Study the drawing (mm; zero at the part's minimum x, y, z) and answer. A direction names the side the tool comes from. Coordinates: 2 decimals unless noted, no trailing zeros. Loops run counter-clockwise (first coordinate to the right, second up) from the corner with the lowest first, then second, coordinate; pieces in that order, holes last. Notation, with made-up numbers: (4.25, -18) -> (57.25, -18) arc R24 cw to (57.25, 16) -> close; hole circle Ø6 at (-9.75, -34.75). An arc over 180 degrees is marked (long way). One line per question, with ' | ' between items.
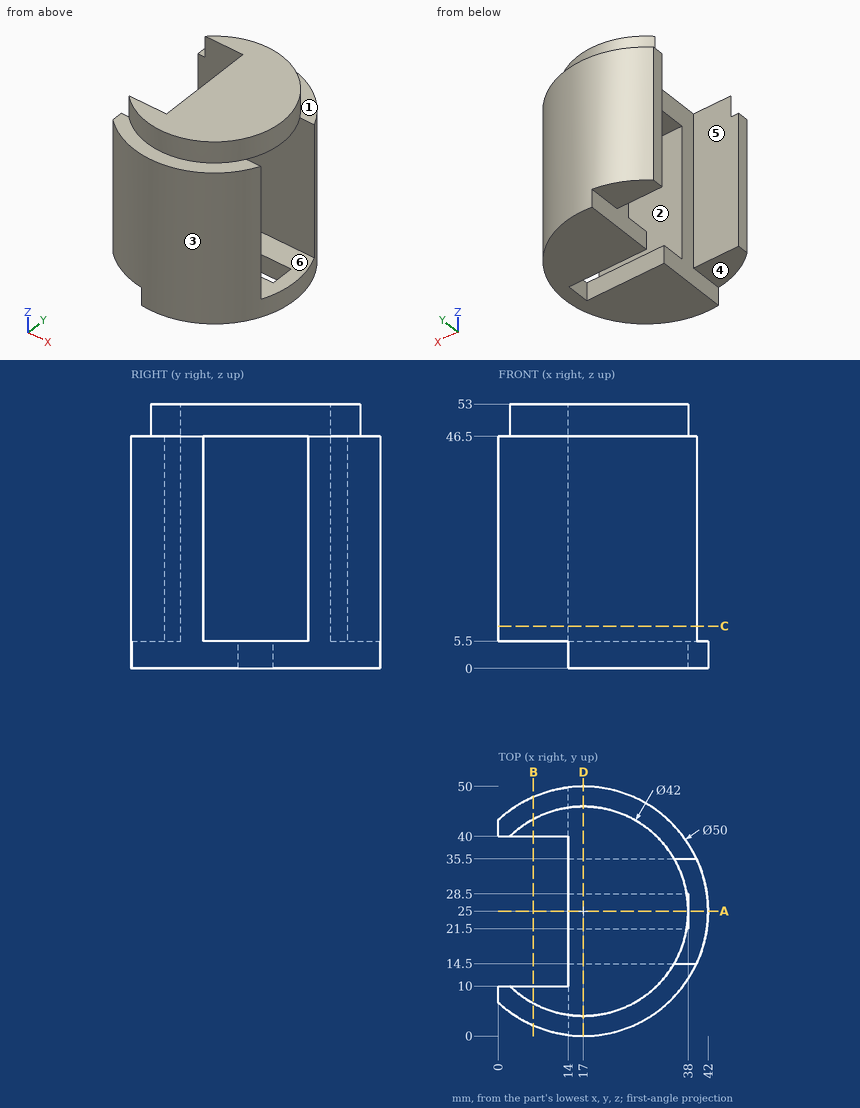
1) Flat-ended cylindrical pins translate along their axes: pin 1 (5 mm diameter, centred on x = 35.5, y = 41.5, fed in from +Z); pin 2 (2 mm diameter, centred on x = 14.5, z = 28.5, fed in from -Y); pin 3 (5 mm diameter, centred on x = 8, y = 3, fed in from -Z). Find the tip coordinate at first contact, or state that the pin passes through.
Check values:
pin 1: stops at z = 46.5 | pin 2: stops at y = 0.05 | pin 3: stops at z = 5.5
2) For the marked faces 4, 5 and 6, determine the directions among +Z, -Z, +X, -X, +Y, -Y from which every point of the face is accessible in a straight line to the end or side of a thin tool.
Check values:
face 4: -Z, -X, +Y, -Y | face 5: +Z, -Z, -X | face 6: +X, -X
3) Find section B-B (x = 7). Write down the section's boundary in (y, z).
Check values:
outline: (2.09, 5.5) -> (10, 5.5) -> (10, 53) -> (6.53, 53) -> (6.53, 46.5) -> (2.09, 46.5) -> close; (40, 5.5) -> (47.91, 5.5) -> (47.91, 46.5) -> (43.47, 46.5) -> (43.47, 53) -> (40, 53) -> close
4) The mould has two halves that part along Y. Classify the marked faces 1, 2 and 3: released by +Y, released by -Y, zero draft, split by the parting line, or undercut.
Check values:
face 1: zero draft | face 2: undercut | face 3: split by the parting line
5) Find the intervals of material crossed by line 1 along Z through (x, y) = (27.5, 16); line 2 along Y through (x, z) = (34, 33.5); line 3 along Y through (x, z) = (13, 27), in increasing order.
Check values:
line 1: z = 0 to 5.5, 46.5 to 53 | line 2: y = 6.67 to 14.5, 35.5 to 43.33 | line 3: y = 0.32 to 10, 40 to 49.68
6) Find section A-A (y = 25). Write down the section's boundary in (x, z).
Check values:
outline: (14, 46.5) -> (38, 46.5) -> (38, 53) -> (14, 53) -> close; (38, 0) -> (42, 0) -> (42, 5.5) -> (38, 5.5) -> close
7) Find section D-D (x = 17). Write down the section's boundary in (y, z).
Check values:
outline: (0, 0) -> (21.5, 0) -> (21.5, 5.5) -> (14.5, 5.5) -> (14.5, 46.5) -> (35.5, 46.5) -> (35.5, 5.5) -> (28.5, 5.5) -> (28.5, 0) -> (50, 0) -> (50, 46.5) -> (46, 46.5) -> (46, 53) -> (4, 53) -> (4, 46.5) -> (0, 46.5) -> close
8) Find section C-C (z = 8.5). Write down the section's boundary in (x, y).
Check values:
outline: (0, 6.67) arc R25 ccw to (39.69, 14.5) -> (14, 14.5) -> (14, 10) -> (0, 10) -> close; (0, 40) -> (14, 40) -> (14, 35.5) -> (39.69, 35.5) arc R25 ccw to (0, 43.33) -> close
